Part model, mm, in its own coordinate system. Coordinates: 2 decimals unless noted, no trailing zeros. Order: outer loops, then holes, each group sorted by start corner. A loop starts at its lowest first (then second) coordinate and runs counter-clockwise, first axis right, second up. Notation, with made-up numbers: M 60,58.25 L 101,58.25 A6 ccw 101,64.25 Z; hole C 56.5,-26.75 d11. An arc over 180 degrees is marked long. Answer in a Markdown table with one row per item. Add a question column.
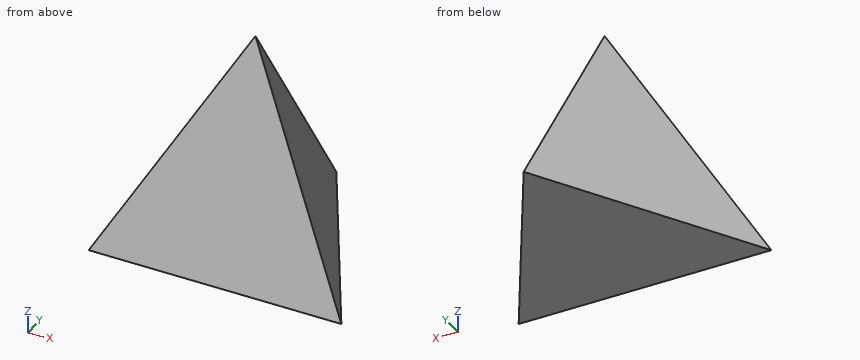
Solid Edge part; units mm, degrees
sketch "Sketch1" plane through (0, 0, 0) normal (0, 0, 1) x (1, 0, 0)
  line L0 (-34.641, -20) -> (34.641, -20)
  line L1 (34.641, -20) -> (0, 40)
  line L2 (0, 40) -> (-34.641, -20)
extrude "Protrusion1" add sketch "Sketch1" along normal up to vertex (60 mm away)
sketch "Sketch2" plane through (0, 0, 0) normal (1, 0, 0) x (0, 1, 0)
  line L0 (-20, 60) -> (-20, 0)
  line L1 (-20, 0) -> (0, 60)
  line L2 (0, 60) -> (-20, 60)
extrude "Cutout1" cut sketch "Sketch2" along normal mid plane 69.282
pattern_circular "Pattern1" count 3 over 360 about axis through (0, 0, 60) along (0, 0, 1) of "Protrusion1"
sketch "Sketch3" plane through (0, 0, 0) normal (1, 0, 0) x (0, 1, 0)
  line L0 (-20, 60) -> (-20, 0)
  line L1 (-20, 0) -> (0, 60)
  line L2 (0, 60) -> (-20, 60)
extrude "Cutout2" cut sketch "Sketch3" along normal mid plane 69.282
pattern_circular "Pattern2" count 3 over 360 about axis through (0, 0, 60) along (0, 0, 1) of "Cutout2"
(1) Slice it at B-B (y = -5). List the corners of the cut face in (x, z), and give its area (3 significant figures).
(2) Slice it at C-C (z = 30). List the corners of the cut face in (x, y).
(3) Slice it at A-A (x = -28). List the corners of the cut face in (y, z), and give its area (3 significant figures).
(4) Drop flat-ended pins along their axis: P1, Ø3, axis at x = 4, z = 9, coming from the +Y side; P2, Ø12, axis at x = 4.5, z = 28, coming from the -Y side; P3, Ø2, axis at x = -3, z = 43, coming from the -Y side; P4, Ø1.5, axis at x = 16, y = 16.5, coming from the -Z side. Give the stop position or say it passes through.
(5) Wall check: line 1 (Y direction, x = 17, z = 10); line 2 (X direction, y = 15.5, z = 28); line 3 (Y direction, x = 5.5, z = 37). Give the ranges that are in metal, low to high.
Computed:
| question | item | result |
|---|---|---|
| 1 | outline | M -25.98,0 L 25.98,0 L 8.66,45 L -8.66,45 Z |
| 1 | area | 1,560 mm^2 |
| 2 | outline | M -17.32,-10 L 17.32,-10 L 0,20 Z |
| 3 | outline | M -20,0 L -8.5,0 L -16.17,11.5 Z |
| 3 | area | 66.2 mm^2 |
| 4 | P1 | stops at y = 29.86 |
| 4 | P2 | stops at y = -12.67 |
| 4 | P3 | stops at y = -6 |
| 4 | P4 | passes through |
| 5 | line 1 | y = -16.67 to 3.89 |
| 5 | line 2 | x = -3.37 to 3.37 |
| 5 | line 3 | y = -7.67 to 5.81 |
